Verification items for the finished model (mm, model axes). A direction names the side the tool comes from. Give positions to 0.01 mm unless a question says otherwise; leave off trailing zeros. Write each loop counter-clockwise with the first axis right and the second up, starting at its lowest first coordinate (ties: lowest second). Pieces come first, ordered by that corner, then holes. Notation, with made-up numbers: M 82.25,48 L 98.25,48 A21 ccw 98.25,56 Z; hole C 34.25,19 d9. An arc over 180 degrees is marked long. Write item = value, one per line.
from build123d import *

# Parameters (mm, degrees)
EXTRUDE_1_DEPTH      = 40
SKETCH_7_W           = 20
SKETCH_7_H           = 8.5
EXTRUDE_5_DEPTH      = 40
SKETCH_8_R           = 1.5
CUT_EXTRUDE_2_DEPTH  = 107.874926901
SKETCH_9_R           = 1.5
CUT_EXTRUDE_3_DEPTH  = 107.874926901
EXTRUDE_6_DEPTH      = 10
EXTRUDE_6_DEPTH_BACK = 40
SKETCH_10_W          = 6
SKETCH_10_H          = 21
SKETCH_11_R          = 2
CUT_EXTRUDE_4_DEPTH  = 109.115678789


with BuildPart() as part:
    # 草图1 → 凸台-拉伸1 (new body)
    with BuildSketch(Plane(origin=(0, 0, 0), x_dir=(1, 0, 0), z_dir=(0, 1, 0))):
        Polygon((0, 0), (90, 0), (90, 6), (30, 6), (30, 27), (90, 27), (90, 33), (0, 33), align=None)
    extrude(amount=EXTRUDE_1_DEPTH)

    # 草图7 → 凸台-拉伸5 (add)
    with BuildSketch(Plane(origin=(0, 40, 0), x_dir=(1, 0, 0), z_dir=(0, 1, 0))):
        with Locations((10, -4.25)):
            Rectangle(SKETCH_7_W, SKETCH_7_H)
    extrude(amount=-EXTRUDE_5_DEPTH)

    # 草图8 → 切除-拉伸2 (cut, through all)
    with BuildSketch(Plane(origin=(0, 0, -33), x_dir=(-1, 0, 0), z_dir=(0, 0, -1))):
        with Locations((-84, 8)):
            Circle(SKETCH_8_R)
        with Locations((-84, 32)):
            Circle(SKETCH_8_R)
        with Locations((-16, 32)):
            Circle(SKETCH_8_R)
        with Locations((-16, 8)):
            Circle(SKETCH_8_R)
    extrude(amount=-CUT_EXTRUDE_2_DEPTH, mode=Mode.SUBTRACT)

    # 草图9 → 切除-拉伸3 (cut, through all)
    with BuildSketch(Plane.XY.offset(8.5)):
        with Locations((4, 32)):
            Circle(SKETCH_9_R)
        with Locations((4, 8)):
            Circle(SKETCH_9_R)
    extrude(amount=-CUT_EXTRUDE_3_DEPTH, mode=Mode.SUBTRACT)

    # 草图10 → 凸台-拉伸6 (add, two sides: drawn at the far end of the back side and taken through both)
    with BuildSketch(Plane(origin=(0, 40, 0), x_dir=(1, 0, 0), z_dir=(0, 1, 0)).offset(-EXTRUDE_6_DEPTH_BACK)):
        with Locations((75, 16.5)):
            Rectangle(SKETCH_10_W, SKETCH_10_H)
    extrude(amount=EXTRUDE_6_DEPTH + EXTRUDE_6_DEPTH_BACK)

    # 草图11 → 切除-拉伸4 (cut, through all)
    with BuildSketch(Plane.XY):
        with Locations((40, 25)):
            Circle(SKETCH_11_R)
    extrude(amount=-CUT_EXTRUDE_4_DEPTH, mode=Mode.SUBTRACT)


solid = part.part
1) Tool access check on faces 1 (the flat face through (84, 20, -6)), 2 (the flat face through (51, 20, -6)), 3 (the flat face through (55, 20, 0)). Record the directions out of +Z, -Z, +X, -X, +Y, -Y that give a thin tool (end or side, any length) a straight path to the whole face; none if there is none.
From the geometry:
face_1 = +X, +Y, -Y
face_2 = +Y, -Y
face_3 = +Z, +X, +Y, -Y
2) Cross-section at D-D on z = -29. Record the boundary of the cut face in (x, y).
From the geometry:
outline = M 0,0 L 90,0 L 90,40 L 0,40 Z; hole C 4,8 d3; hole C 4,32 d3; hole C 16,8 d3; hole C 16,32 d3; hole C 40,25 d4; hole C 84,8 d3; hole C 84,32 d3
3) Cross-section at C-C on y = 17.5. Record the boundary of the cut face in (x, z).
From the geometry:
outline = M 0,-33 L 90,-33 L 90,-27 L 78,-27 L 78,-6 L 90,-6 L 90,0 L 20,0 L 20,8.5 L 0,8.5 Z; hole M 30,-27 L 72,-27 L 72,-6 L 30,-6 Z
4) Material ranges on probe 1 along Y at (x, z) = (4, -16.5); probe 2 along Z at (x, y) = (56.5, 33); probe 3 along Y at (x, z) = (40, -29.85), recorded low to high. Write a range as from..to.
From the geometry:
probe_1 = 0..6.5, 9.5..30.5, 33.5..40
probe_2 = -33..-27, -6..0
probe_3 = 0..23, 27..40
5) Draft check along Z on faces 4 (the flat face through (30, 20, -16)), 5 (the cylindrical face through (40, 23, -3)), 6 (the flat face through (10, 20, 8.5)). Enter one of: +Z half, -Z half, draft (parallel to the pull), parting line (faces both ways), or undercut.
From the geometry:
face_4 = undercut
face_5 = draft
face_6 = +Z half
6) Cross-section at B-B on x = 16. Record the boundary of the cut face in (y, z), plus the area to 3 significant figures.
From the geometry:
outline = M 0,-33 L 6.5,-33 L 6.5,8.5 L 0,8.5 Z; M 9.5,-33 L 30.5,-33 L 30.5,8.5 L 9.5,8.5 Z; M 33.5,-33 L 40,-33 L 40,8.5 L 33.5,8.5 Z
area = 1,410 mm^2
7) Cross-section at A-A on z = -11.5. Record the boundary of the cut face in (x, y).
From the geometry:
outline = M 0,0 L 30,0 L 30,40 L 0,40 Z; M 72,0 L 78,0 L 78,50 L 72,50 Z; hole C 4,8 d3; hole C 4,32 d3; hole C 16,8 d3; hole C 16,32 d3
8) Depth check by flat-ended pin: P1, Ø20, axis at x = 57.5, y = 23, coming from the +Z side; P2, Ø8, axis at x = 43, z = -11.5, coming from the +Y side; P3, Ø17, axis at y = 28.5, z = -18, coming from the +X side; P4, Ø5, axis at x = 74.5, y = 43.5, coming from the +Z side. Enter the tip coordinate at first touch or a pass-through.
From the geometry:
P1 = 0
P2 = through
P3 = 78
P4 = -6
